Input: part model. Units: mm. Frame: model coordinates. A direction names the side the tool comes from. Coordinates: 2 decimals unless noted, no trailing zeros. Order: outer loops, then holes, each group sorted by start corner. A loop starts at its lowest first (then second) coordinate and runs counter-clockwise, first axis right, second up. Notation, with made-up numbers: (19.25, 67) -> (68.25, 67) arc R17 cw to (68.25, 95) -> close; hole circle Ø9 at (40.5, 25). An arc over 180 degrees is marked (long way). One line per question, with ' | ' between items.
```python
from build123d import *

# Parameters (mm, degrees)
F0_W         = 177.8
F0_H         = 127
F1_DEPTH     = 12.7
F2_R         = 3.175
F3_DEPTH     = 127
F6_W         = 13.4703841816
F6_H         = 6.35
F7_DEPTH     = 1.27
F8_R         = 2.54
F9_T1_DEPTH  = 10.16
F9_T3_DEPTH  = 7.62
F9_T5_DEPTH  = 10.1599999705
F9_S9_W      = 2.54
F9_S9_H      = 2.54
F9_T10_DEPTH = 2.54
F9_S15_W     = 2.54
F9_S15_H     = 2.54
F9_T16_DEPTH = 2.54
F9_T22_DEPTH = 171.4500000295
F9_S23_R     = 3.175
F9_T24_DEPTH = 87
F9_T28_DEPTH = 120.65
F9_S29_R     = 3.175
F9_T30_DEPTH = 62


# Not quite as in the source:
# - a fillet or chamfer that OpenCascade refuses, or shapes differently, is made with other operations: its cross-section is extruded or revolved along the edge and cut away or added


with BuildPart() as f1:
    # F0 (on Top) → F1 (new body)
    with BuildSketch(Plane.XY):
        Rectangle(F0_W, F0_H)
    extrude(amount=F1_DEPTH)

    # F2 (on Top) → F3 (join)
    with BuildSketch(Plane.XY):
        with Locations((76.2, -60.325)):
            Circle(F2_R)
        with Locations((85.725, -50.8)):
            Circle(F2_R)
    extrude(amount=-F3_DEPTH)

    # F6 (on face) → F7 (join, symmetric)
    with BuildSketch(Plane(origin=(68.2625, -68.2625, 0), x_dir=(0.7071067812, 0.7071067812, 0), z_dir=(0.7071067812, -0.7071067812, 0))):
        with Locations((17.9605122421, -22.225)):
            Rectangle(F6_W, F6_H)
        with Locations((17.9605122421, -47.625)):
            Rectangle(F6_W, F6_H)
        Polygon((11.2253201513, -76.2), (24.6957043329, -76.2), (24.6957043329, -69.85), (11.2336926315, -69.85), (11.2253201513, -69.85), align=None)
        with Locations((17.9605122421, -98.425)):
            Rectangle(F6_W, F6_H)
        with Locations((17.9605122421, -123.825)):
            Rectangle(F6_W, F6_H)
    extrude(amount=F7_DEPTH, both=True)

    # F8
    f8_edges = [f1.edges().sort_by_distance(p)[0] for p in [
        (0, -63.5, 12.7),
        (88.9, 0, 12.7),
        (0, 63.5, 12.7),
        (-88.9, 0, 12.7),
    ]]
    fillet(f8_edges, radius=F8_R)

    # F9: fillet of radius 2.54 on 3 edges, made by hand

    # F9_s2 → F9_t1 (cut)
    with BuildSketch(Plane.XZ.offset(50.8)):
        with BuildLine():
            ThreePointArc((86.36, 0), (88.1560512242, 0.7439487758), (88.9, 2.54))
            Line((88.9, 2.54), (88.9, 0))
            Line((88.9, 0), (86.36, 0))
        make_face()
    extrude(amount=F9_T1_DEPTH, mode=Mode.SUBTRACT)

    # F9_s4 → F9_t3 (cut)
    with BuildSketch(Plane.XY.offset(2.54)):
        with BuildLine():
            ThreePointArc((86.36, -63.5), (88.1560512242, -62.7560512242), (88.9, -60.96))
            Line((88.9, -60.96), (88.9, -63.5))
            Line((88.9, -63.5), (86.36, -63.5))
        make_face()
    extrude(amount=F9_T3_DEPTH, mode=Mode.SUBTRACT)

    # F9_s6 → F9_t5 (cut)
    with BuildSketch(Plane.YZ.offset(76.2000000295)):
        with BuildLine():
            ThreePointArc((-63.5, 2.54), (-62.7560512242, 0.7439487758), (-60.96, 0))
            Line((-60.96, 0), (-63.5, 0))
            Line((-63.5, 0), (-63.5, 2.54))
        make_face()
    extrude(amount=F9_T5_DEPTH, mode=Mode.SUBTRACT)


with BuildPart() as f9_tool8:
    # F9_s9 → F9_t10 (new body)
    with BuildSketch(Plane.XZ.offset(60.96)):
        with Locations((87.63, 11.43)):
            Rectangle(F9_S9_W, F9_S9_H)
    extrude(amount=F9_T10_DEPTH)

    # F9_s11 → F9_t12 (revolve, cut)
    with BuildSketch(Plane(origin=(86.36, -60.96, 10.16), x_dir=(-0.7071067812, 0, -0.7071067812), z_dir=(-0.7071067812, 0, 0.7071067812))):
        with BuildLine():
            ThreePointArc((0, -2.54), (2.54, 0), (0, 2.54))
            Line((0, 2.54), (0, -2.54))
        make_face()
    revolve(axis=Axis((86.36, -60.96, 10.16), (0, -1, 0)), mode=Mode.SUBTRACT)


with BuildPart() as f1_1:
    add(f1.part)

    # F9_t7: cut F9_tool8
    add(f9_tool8.part, mode=Mode.SUBTRACT)


with BuildPart() as f9_tool14:
    # F9_s15 → F9_t16 (new body)
    with BuildSketch(Plane.XZ.offset(60.96)):
        with Locations((87.63, 1.27)):
            Rectangle(F9_S15_W, F9_S15_H)
    extrude(amount=F9_T16_DEPTH)

    # F9_s17 → F9_t18 (revolve, cut)
    with BuildSketch(Plane(origin=(86.36, -60.96, 2.54), x_dir=(-0.7071067812, 0, 0.7071067812), z_dir=(0.7071067812, 0, 0.7071067812))):
        with BuildLine():
            ThreePointArc((0, -2.54), (2.54, 0), (0, 2.54))
            Line((0, 2.54), (0, -2.54))
        make_face()
    revolve(axis=Axis((86.36, -60.96, 2.54), (0, -1, 0)), mode=Mode.SUBTRACT)


with BuildPart() as f1_2:
    add(f1_1.part)

    # F9_t13: cut F9_tool14
    add(f9_tool14.part, mode=Mode.SUBTRACT)


with BuildPart() as f9_tool20:
    # F9_s21 → F9_t22 (new body)
    with BuildSketch(Plane.YZ.offset(-95.25)):
        with BuildLine():
            ThreePointArc((-63.5, 2.54), (-62.7560512242, 0.7439487758), (-60.96, 0))
            Line((-60.96, 0), (-63.5, 0))
            Line((-63.5, 0), (-63.5, 2.54))
        make_face()
    extrude(amount=F9_T22_DEPTH)

    # F9_s23 → F9_t24 (cut, symmetric)
    with BuildSketch(Plane.XY.offset(1.3)):
        with Locations((76.2, -60.325)):
            Circle(F9_S23_R)
    extrude(amount=F9_T24_DEPTH, both=True, mode=Mode.SUBTRACT)


with BuildPart() as f1_3:
    add(f1_2.part)

    # F9_t19: cut F9_tool20
    add(f9_tool20.part, mode=Mode.SUBTRACT)


with BuildPart() as f9_tool26:
    # F9_s27 → F9_t28 (new body)
    with BuildSketch(Plane.XZ.offset(50.8)):
        with BuildLine():
            ThreePointArc((86.36, 0), (88.1560512242, 0.7439487758), (88.9, 2.54))
            Line((88.9, 2.54), (88.9, 0))
            Line((88.9, 0), (86.36, 0))
        make_face()
    extrude(amount=-F9_T28_DEPTH)

    # F9_s29 → F9_t30 (cut, symmetric)
    with BuildSketch(Plane.XY.offset(1.3)):
        with Locations((85.725, -50.8)):
            Circle(F9_S29_R)
    extrude(amount=F9_T30_DEPTH, both=True, mode=Mode.SUBTRACT)


with BuildPart() as f1_4:
    add(f1_3.part)

    # F9_t25: cut F9_tool26
    add(f9_tool26.part, mode=Mode.SUBTRACT)

    # F10: F1 across plane


with BuildPart() as f1_5:
    add(f1_4.part)
    add(f1_4.part.mirror(Plane.YZ))

    # F11: F1 across plane


with BuildPart() as f1_6:
    add(f1_5.part)
    add(f1_5.part.mirror(Plane.XZ))


solid = f1_6.part
```
1. Cut plane A-A, the plane z = -21.5. Return loops of the section in (x, y) (3 decimals).
Recorded:
outline: (-84.565, -53.756) -> (-79.156, -59.165) arc R3.175 ccw (long way) to (-77.36, -57.369) -> (-82.769, -51.96) arc R3.175 ccw (long way) to start; (-84.565, 53.756) arc R3.175 ccw (long way) to (-82.769, 51.96) -> (-77.36, 57.369) arc R3.175 ccw (long way) to (-79.156, 59.165) -> close; (77.36, -57.369) arc R3.175 ccw (long way) to (79.156, -59.165) -> (84.565, -53.756) arc R3.175 ccw (long way) to (82.769, -51.96) -> close; (77.36, 57.369) -> (82.769, 51.96) arc R3.175 ccw (long way) to (84.565, 53.756) -> (79.156, 59.165) arc R3.175 ccw (long way) to start
2. Mould query, pull axis Y, two halves, no side actions, for faces 1 (the face through (82, 56, -127)), 2 (the face through (-81, 56, -120.65)). Classes: released by +Y, released by -Y, zero draft, split by the parting line, or undercut.
Recorded:
face 1: zero draft | face 2: undercut
3. Cut plane C-C, the plane x = 13.5. Return loops of the section in (y, z).
Recorded:
outline: (-63.5, 0) -> (63.5, 0) -> (63.5, 10.16) arc R2.54 ccw to (60.96, 12.7) -> (-60.96, 12.7) arc R2.54 ccw to (-63.5, 10.16) -> close
4. Cut plane B-B, the plane y = -16. Return loops of the section in (x, z).
Recorded:
outline: (-88.9, 0) -> (88.9, 0) -> (88.9, 10.16) arc R2.54 ccw to (86.36, 12.7) -> (-86.36, 12.7) arc R2.54 ccw to (-88.9, 10.16) -> close
5. Access query for faces 3 (the face through (81, -56, -120.65)), 4 (the face through (-80.03, -54.7, -47.58)). Directions: +Z, -Z, +X, -X, +Y, -Y. A direction counts if a zero-diameter tool reaches every point of the face in a straight line with its end or side. Return the directions, or none.
Recorded:
face 3: none | face 4: -Z
6. Ray query, line 1 (Z direction, x = 47, y = 47); line 2 (X direction, y = 51, z = -87); line 3 (X direction, y = 50, z = -74). Return the intervals inside material, ascending. Write a range as [from, to].
Recorded:
line 1: z = [0, 12.7] | line 2: x = [-88.89, -82.56], [82.56, 88.89] | line 3: x = [-88.8, -82.65], [82.65, 88.8]
7. Pin query (flat end, axial travel): pin 1 Ø1.5 at (x, y) = (-26, -17) entering from -Z; pin 2 Ø6 at (y, z) = (-46, -10.5) entering from +X. Return the tip coordinate at first contact, or that it passes through.
Recorded:
pin 1: stops at z = 0 | pin 2: stops at x = 88.34
